```python
from build123d import *

# Parameters (mm, degrees)
SKETCH1_R           = 2
BOSS_EXTRUDE1_DEPTH = 3
SKETCH3_R           = 1.5
SKETCH4_W           = 8
SKETCH4_H           = 1.5
CUT_EXTRUDE1_DEPTH  = 10
CUT_EXTRUDE2_DEPTH  = 10


with BuildPart() as part:
    # Sketch1 → Boss-Extrude1 (new body)
    with BuildSketch(Plane(origin=(0, 0, 0), x_dir=(1, 0, 0), z_dir=(0, 1, 0))):
        with BuildLine():
            Line((0, 0), (0, 20))
            Line((0, 20), (-8, 20))
            Line((-8, 20), (-8, -8))
            Line((-8, -8), (10, -8))
            Line((10, -8), (10, -6))
            Line((10, -6), (4, -6))
            ThreePointArc((4, -6), (2, -4), (4, -2))
            Line((4, -2), (10, -2))
            Line((10, -2), (10, 0))
            Line((10, 0), (0, 0))
        make_face()
        with Locations((-4, -4)):
            Circle(SKETCH1_R, mode=Mode.SUBTRACT)
    extrude(amount=BOSS_EXTRUDE1_DEPTH)

    # Sweep1: sweep along a path in Sketch2
    with BuildLine(Plane(origin=(0, 1.5, 0), x_dir=(1, 0, 0), z_dir=(0, 1, 0))) as sweep1_path:
        Line((-8, 16), (-70.679491924, 16))
        ThreePointArc((-70.679491924, 16), (-79.339745962, 21), (-79.339745962, 31))
        Line((-79.339745962, 31), (-6.839745962, 156.573683549))
    # Sketch3 → Sweep1 (sweep)
    with BuildSketch(Plane.ZY.offset(8)):
        with Locations((-15.996391196, 1.5)):
            Circle(SKETCH3_R)
    sweep(path=sweep1_path.line)

    # Sketch4 → Cut-Extrude1 (cut)
    with BuildSketch(Plane(origin=(0, 0, 0), x_dir=(-1, 0, 0), z_dir=(0, 0, -1))):
        with Locations((-6, 2.25)):
            Rectangle(SKETCH4_W, SKETCH4_H)
    extrude(amount=-CUT_EXTRUDE1_DEPTH, mode=Mode.SUBTRACT)

    # Sketch5 → Cut-Extrude2 (cut)
    with BuildSketch(Plane.ZY.offset(8)):
        with BuildLine():
            Line((-15.996391196, 3), (-20, 3))
            Line((-20, 3), (-20, 0))
            Line((-20, 0), (-15.996391196, 0))
            ThreePointArc((-15.996391196, 0), (-17.496391196, 1.5), (-15.996391196, 3))
        make_face()
    extrude(amount=-CUT_EXTRUDE2_DEPTH, mode=Mode.SUBTRACT)


solid = part.part
```
For this review, take the finished solid that the model builds, in its own axes (mm). A direction names the side the tool comes from. Round coordinates to 2 decimals unless told otherwise and drop trailing zeros. Loops run counter-clockwise (first coordinate to the right, second up) from the corner with the lowest first, then second, coordinate; pieces in that order, holes last.
(1) We need section A-A (x = -4). Give the boundary of the cut face in (y, z), plus the area to 3 significant figures.
Returned:
outline: (0, -16) arc R1.5 ccw to (3, -16) - (3, 2) - (0, 2) - close; (0, 6) - (3, 6) - (3, 8) - (0, 8) - close
area: 63.5 mm2
(2) Tool access review of faces 1 (the flat face through (6, 1.5, 7)), 2 (the flat face through (0, 1, -9)), 3 (the flat face through (-1, 0, -1)): name each direction out of +Z, -Z, +X, -X, +Y, -Y from which nothing blocks a thin tool from reaching the whole face with its end or side.
Returned:
face 1: +Z, -Z, +X, +Y
face 2: -Z, +X, +Y, -Y
face 3: +Z, -Z, +X, -X, -Y
(3) Wall thickness on line 1 along X through (y, z) = (0.75, 4); line 2 along Z through (x, y) = (-4, 1.55); line 3 along Z through (x, y) = (-4, 2.05): over which ranges is each line inside the solid? List them lowest first.
Returned:
line 1: x = -8 to -6, -2 to 2
line 2: z = -17.5 to 2, 6 to 8
line 3: z = -17.39 to 2, 6 to 8
(4) Clearance check with flat-ended pins moving along their axes: P1, Ø3, axis at x = 4, z = 1, coming from the +Y side; P2, Ø0.9, axis at y = 1, z = -5.5, coming from the +X side; P3, Ø0.9, axis at y = 1.5, z = -0.5, coming from the -X side. State where each tip first meets the part, or that it passes through.
Returned:
P1: stops at y = 1.5
P2: stops at x = 0
P3: stops at x = -8
(5) We need section B-B (y = 2.4). Give the boundary of the cut face in (x, z).
Returned:
outline: (-80.38, -31.6) - (-7.88, -157.18) - (-5.8, -155.98) - (-78.3, -30.4) arc R8.8 cw to (-70.68, -17.2) - (0, -17.2) - (0, 0) - (2, 0) - (2, 8) - (-8, 8) - (-8, -14.8) - (-70.68, -14.8) arc R11.2 ccw to start; hole circle Ø4 at (-4, 4)
(6) Mouldability with a two-part tool opening along Z and no side actions: class faces 4 (the flat face through (-1, 1, 8)), 5 (the cylindrical face through (-5.6, 1.5, 5.2)), 6 (the flat face through (4, 1, 0)) as released by +Z, released by -Z, zero draft, split by the parting line, or undercut.
Returned:
face 4: released by +Z
face 5: undercut
face 6: released by -Z
